Part print with two shaded views. Sizes in mm from the minimum x, y, z corner. A direction names the side the tool comes from. Coordinates: 2 decimals unless noted, no trailing zeros. Order: outer loops, then holes, each group sorted by start corner. A loop starts at its lowest first (then second) coordinate and runs counter-clockwise, first axis right, second up. Notation, with made-up numbers: (56, 32.25) - (109, 32.25) arc R36 ccw to (109, 69.25) - close; hole circle Ø1 at (68, 13.25). An arc over 180 degrees is marked (long way). Write each question's results on one line, items separated by ' | '. Start each with the question number.
Q1. Band-saw the part on C-C, the plane z = 32.5. Write the cut outline in (x, y), then the cut area to 3 significant figures.
Q2. Which spindle directions (+Z, -Z, +X, -X, +Y, -Y) get a long thin tool onto all of the face, cutting with end or side? Do the marked faces 1, 2 and 3. Say none if no direction does.
Q3. Band-saw the part on B-B, the plane y = 13. Write the cut outline in (x, z), then the cut area to 3 significant figures.
Q4. Pin check, flat tips, straight feed: P1, Ø8, axis at x = 4.5, z = 7.5, coming from the +Y side; P2, Ø2, axis at y = 21, z = 15.5, coming from the -X side; P3, Ø8, axis at y = 13, z = 32.5, coming from the +X side; P4, Ø3.5, axis at x = 22, z = 31.5, coming from the +Y side. Stop position of each tip, or through.
Q5. Pull direction Y, two halves, no side cores. Call the marked faces 4, 5 and 6: released by +Y, released by -Y, zero draft, split by the parting line, or undercut.
Q6. Band-saw the part on D-D, the plane z = 24.5. Write the cut outline in (x, y).
Q7. Band-saw the part on A-A, the plane x = 16.5. Write the cut outline in (y, z), then the cut area to 3 significant figures.
Q8. Wall check: probe 1 along Y at (x, z) = (15, 19.5); probe 2 along Z at (x, y) = (18.6, 13); probe 3 along Y at (x, z) = (19.35, 32.5). Give the ranges that are in metal, low to high.
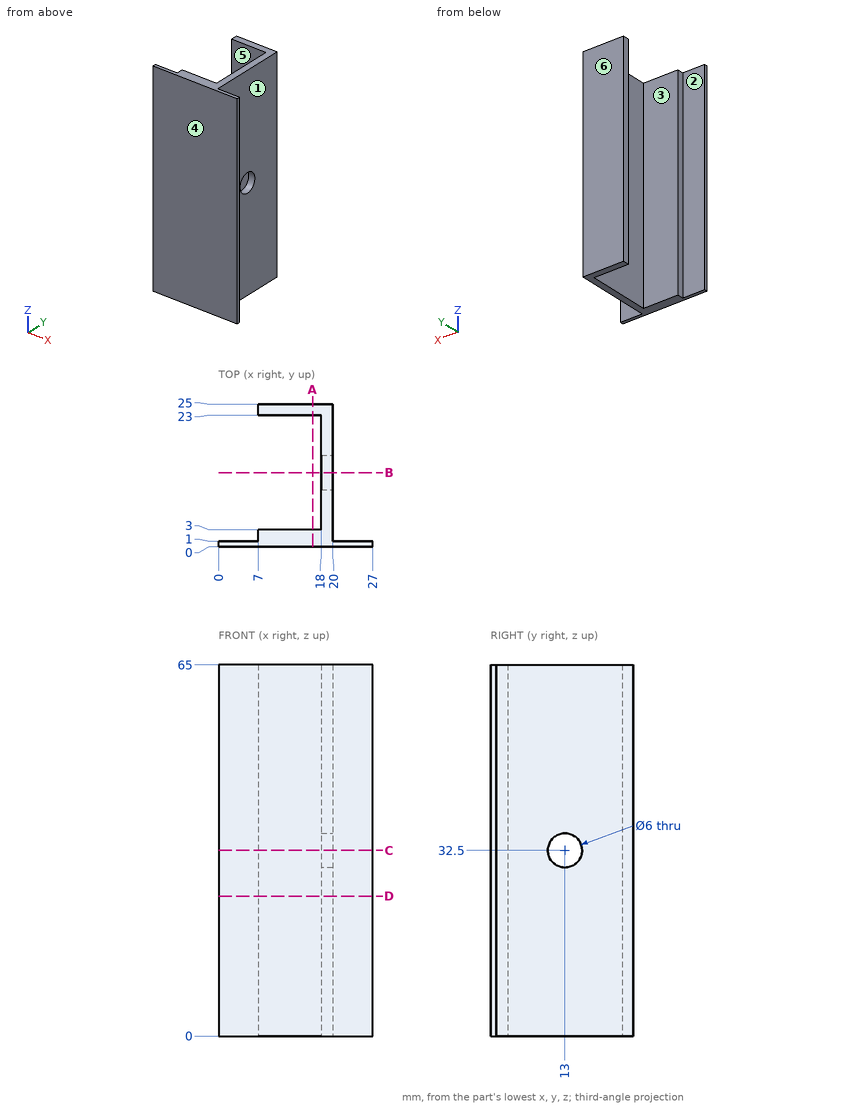
Results below:
1) outline: (0, 0) - (27, 0) - (27, 1) - (20, 1) - (20, 10) - (18, 10) - (18, 3) - (7, 3) - (7, 1) - (0, 1) - close; (7, 23) - (18, 23) - (18, 16) - (20, 16) - (20, 25) - (7, 25) - close | area: 107 mm²
2) face 1: +Z, -Z, +X, +Y | face 2: +Z, -Z, -X, +Y | face 3: +Z, -Z, -X
3) outline: (18, 0) - (20, 0) - (20, 29.5) - (18, 29.5) - close; (18, 35.5) - (20, 35.5) - (20, 65) - (18, 65) - close | area: 118 mm²
4) P1: stops at y = 25 | P2: stops at x = 18 | P3: stops at x = 20 | P4: stops at y = 1
5) face 4: released by -Y | face 5: undercut | face 6: released by +Y
6) outline: (0, 0) - (27, 0) - (27, 1) - (20, 1) - (20, 25) - (7, 25) - (7, 23) - (18, 23) - (18, 3) - (7, 3) - (7, 1) - (0, 1) - close
7) outline: (0, 0) - (3, 0) - (3, 65) - (0, 65) - close; (23, 0) - (25, 0) - (25, 65) - (23, 65) - close | area: 325 mm²
8) probe 1: y = 0 to 3, 23 to 25 | probe 2: z = 0 to 29.5, 35.5 to 65 | probe 3: y = 0 to 10, 16 to 25
